Can you work these out from the model? Positions are in its coordinate system, mm. Give positions to 0.01 mm unless a question says otherwise; leave off trailing zeros. Order: outer loops, then holes, each group sorted by start corner. A loop starts at its lowest first (then second) coordinate and runs counter-clockwise, first axis right, second up. Notation, with made-up numbers: (45, -29) - (50, -29) arc R15 ccw to (50, 0) - close; hole circle Ø9 at (74, -31.5). An arc over 180 degrees is marked (long way). One line per question, with ' | ' between items.
Autodesk Inventor part; units mm, degrees
ref_plane "YZ Plane" through (0, 0, 0) normal (1, 0, 0) x (0, 1, 0)
ref_plane "XZ Plane" through (0, 0, 0) normal (0, 1, 0) x (-1, 0, 0)
ref_plane "XY Plane" through (0, 0, 0) normal (0, 0, 1) x (1, 0, 0)
sketch "Skizze1" plane through (0, 0, 0) normal (0, 0, 1) x (1, 0, 0)
  line L0 (-43, 59) -> (43, 59)
  line L1 (43, 59) -> (43, -59)
  line L2 (43, -59) -> (-43, -59)
  line L3 (-43, -59) -> (-43, 59)
  point P0 (0, 0)
  point P1 (0, 59)
  point P2 (-43, 0)
  dimension "d0" = 86
  dimension "d1" = 118
extrude "Extrusion1" add sketch "Skizze1" against normal blind 14.9
sketch "Skizze2" plane through (0, 0, -14.9) normal (0, 0, -1) x (-1, 0, 0)
  line L0 (-43, -59) -> (43, -59)
  point P0 (0, 0)
  point P1 (-24, 0)
  point P2 (24, 0)
  point P3 (24, -36)
  point P4 (-24, -36)
  dimension "d4" = 36
  dimension "d5" = 48
  dimension "d6" = 23
  dimension "d7" = 24
hole "Bohrung1" at (24, 0, -14.9) at (-24, 0, -14.9) at (-24, -36, -14.9) at (24, -36, -14.9) direction (0, 0, 1) diameter 3.242 depth 11.8 tip angle 118
sketch "Skizze3" plane through (0, 0, 0) normal (0, 0, 1) x (1, 0, 0)
  line L0 (-24, 44) -> (24, 44)
  line L1 (28, 40) -> (28, -40)
  line L2 (24, -44) -> (-24, -44)
  line L3 (-28, -40) -> (-28, 40)
  arc A0 (-28, -40) -> (-24, -44) centre (-24, -40) ccw
  arc A1 (-24, 44) -> (-28, 40) centre (-24, 40) ccw
  arc A2 (28, 40) -> (24, 44) centre (24, 40) ccw
  arc A3 (24, -44) -> (28, -40) centre (24, -40) ccw
  line L4 (43, -59) -> (43, 59)
  line L5 (-43, 59) -> (-43, -59)
  line L6 (43, 59) -> (-43, 59)
  line L7 (-43, -59) -> (43, -59)
  point P0 (0, 0)
  dimension "d15" = 4
  dimension "d16" = 15
  dimension "d17" = 15
  dimension "d18" = 15
  dimension "d19" = 15
sketch "Skizze4" plane through (0, 0, 0) normal (1, 0, 0) x (0, 1, 0)
  arc A0 (-44, 0) -> (-67, -8.688) centre (-44, -34.7882) ccw
  line L0 (59, 0) -> (-59, 0)
  line L1 (-44, 0) -> (-67, 0)
  line L2 (-67, 0) -> (-67, -8.688)
  line L3 (-59, 0) -> (-59, -14.9)
  line L4 (59, -14.9) -> (-59, -14.9)
  point P0 (0, 0)
  point P1 (-59, -3.4)
  dimension "d20" = 23
  dimension "d21" = 11.5
sweep "Sweeping1" cut profiles "Skizze4" path "Skizze3" path curves L2 A3 L1 A2 L0 A1 L3 A0
sketch "Skizze5" plane through (0, 0, 0) normal (0, 1, 0) x (-1, 0, 0)
  line L0 (24, 0) -> (-24, 0)
  line L1 (-43, -3.4) -> (-43, -8.5741)
  line L2 (-43, -8.5741) -> (-43, -14.9)
  line L3 (-43, -8.5741) -> (-43, -14.9)
  line L4 (-43, -8.5741) -> (-43, -3.4)
  line L5 (43, -8.5741) -> (43, -3.4)
  line L6 (43, -3.4) -> (43, -8.5741)
  line L7 (43, -8.5741) -> (43, -14.9)
  line L8 (43, -8.5741) -> (43, -14.9)
  arc A0 (43, -3.4) -> (-43, -3.4) centre (0, -273.6118) ccw
  line L9 (43, -3.4) -> (43, 1)
  line L10 (43, 1) -> (-43, 1)
  line L11 (-43, 1) -> (-43, -3.4)
  point P0 (0, 0)
  point P1 (43, -5.987)
  point P2 (-43, -5.987)
  dimension "d24" = 1
extrude "Extrusion2" cut sketch "Skizze5" along normal through all both and the other way through all
equation "\"d17\" = d16"
properties part number "kühlblock" material "Aluminium 6061"
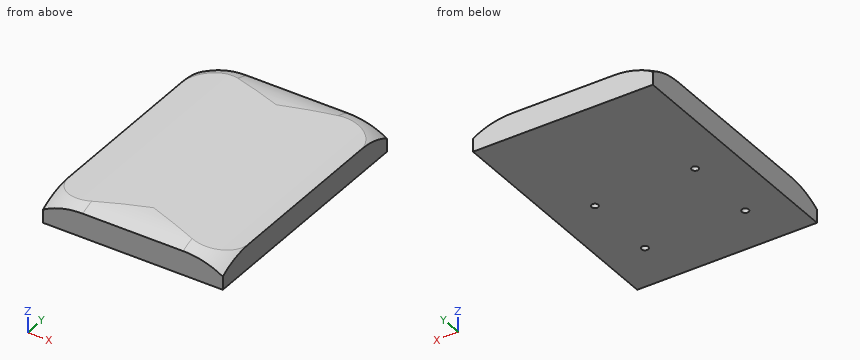
(1) Will these pins go through, and if not, where does the flat tip stop? pin 1 (5 mm diameter, centred on x = 24, y = 0, fed in from +Z); pin 2 (12 mm diameter, centred on x = 14.5, y = 16.5, fed in from +Z); pin 3 (3 mm diameter, centred on x = 14.5, y = 32, fed in from +Z).
Answer below:
pin 1: z = -0.85 | pin 2: z = -0.13 | pin 3: z = -0.31
(2) Imagine slicing it at A-A (y = -4). List the corners of the cut face in (x, z) for me, and give its area (3 significant figures).
Answer below:
outline: (-43, -14.9) - (43, -14.9) - (43, -3.4) arc R273.61 ccw to (-43, -3.4) - close | area: 1,180 mm^2
(3) Imagine slicing it at B-B (x = 19). List the corners of the cut face in (y, z) for me, and give its area (3 significant figures).
Answer below:
outline: (-59, -14.9) - (59, -14.9) - (59, -3.4) arc R34.79 ccw to (50.75, -0.66) - (-50.75, -0.66) arc R34.79 ccw to (-59, -3.4) - close | area: 1,660 mm^2
(4) Imagine slicing it at C-C (x = -12). List the corners of the cut face in (y, z) for me, and give its area (3 significant figures).
Answer below:
outline: (-59, -14.9) - (59, -14.9) - (59, -3.4) arc R34.79 ccw to (48.27, -0.26) - (-48.27, -0.26) arc R34.79 ccw to (-59, -3.4) - close | area: 1,700 mm^2
(5) If I drill on line 1 (Y direction, x = -24, z = -11.75); line 2 (X direction, y = -36, z = -9.25); line 3 (Z direction, x = 30, y = 16), over which ranges is the centre line in solid material (lowest first)?
Answer below:
line 1: -59 to -37.62, -34.38 to -1.62, 1.62 to 59 | line 2: -43 to -25.62, -22.38 to 22.38, 25.62 to 43 | line 3: -14.9 to -1.65
